Autodesk Inventor part; units mm, degrees
ref_plane "YZ Plane" through (0, 0, 0) normal (1, 0, 0) x (0, 1, 0)
ref_plane "XZ Plane" through (0, 0, 0) normal (0, 1, 0) x (-1, 0, 0)
ref_plane "XY Plane" through (0, 0, 0) normal (0, 0, 1) x (1, 0, 0)
sketch "Sketch1" plane through (0, 0, 0) normal (0, 0, 1) x (1, 0, 0)
  line L0 (-22.85, 10.65) -> (22.85, 10.65)
  line L1 (22.85, 10.65) -> (22.85, -10.65)
  line L2 (22.85, -10.65) -> (-22.85, -10.65)
  line L3 (-22.85, -10.65) -> (-22.85, 10.65)
  line L4 (0, 0) -> (0, 10.65) construction
  line L5 (0, 0) -> (0, -10.65) construction
  line L6 (0, 0) -> (22.85, 0) construction
  line L7 (0, 0) -> (-22.85, 0) construction
  dimension "d0" = 45.7
  dimension "d1" = 21.3
extrude "Extrusion1" add sketch "Sketch1" along normal blind 1.75
sketch "Sketch2" plane through (0, 0, 1.75) normal (0, 0, 1) x (1, 0, 0)
  line L0 (22.85, 10.65) -> (22.85, -10.65)
  line L1 (-22.85, 10.65) -> (22.85, 10.65)
  line L2 (22.85, -10.65) -> (-22.85, -10.65)
  point P0 (-20.35, -8.15)
  point P1 (20.35, 8.15)
  dimension "d4" = 2.5
  dimension "d5" = 2.5
  dimension "d6" = 2.5
  dimension "d7" = 2.5
hole "Hole1" at (-20.35, -8.15, 1.75) at (20.35, 8.15, 1.75) direction (0, 0, -1) diameter 3.1 end through all
properties part number "Parallax_Ping_PCB" material "Phenolic"
Geometry check sheet. Reference: the model listing, model coordinates, mm. Give positions to 0.01 mm unless a question says otherwise; leave off trailing zeros. Order: outer loops, then holes, each group sorted by start corner. A loop starts at its lowest first (then second) coordinate and runs counter-clockwise, first axis right, second up. Notation, with made-up numbers: (10.25, 32) - (66.25, 32) arc R24 cw to (66.25, 55) - close; hole circle Ø10 at (-9.5, -18). An arc over 180 degrees is marked (long way). Use one line per item in the form item = value.
1) Sectioned sample at B-B (z = 0.4). Record the boundary of the cut face in (x, y).
Working result:
outline = (-22.85, -10.65) - (22.85, -10.65) - (22.85, 10.65) - (-22.85, 10.65) - close; hole circle Ø3.1 at (-20.35, -8.15); hole circle Ø3.1 at (20.35, 8.15)
2) Sectioned sample at C-C (x = 20.35). Record the boundary of the cut face in (y, z), and give its area (4 significant figures).
Working result:
outline = (-10.65, 0) - (6.6, 0) - (6.6, 1.75) - (-10.65, 1.75) - close; (9.7, 0) - (10.65, 0) - (10.65, 1.75) - (9.7, 1.75) - close
area = 31.85 mm^2
3) Draft check along Y on faces 1 (the face through (0, 10.65, 1)), 2 (the face through (0, -10.65, 1)), 3 (the face through (21.29, 9.38, 0.86)). Enter one of: released by +Y, released by -Y, zero draft, split by the parting line, or undercut.
Working result:
face_1 = released by +Y
face_2 = released by -Y
face_3 = undercut
4) Material ranges on probe 1 along X at (y, z) = (-8.15, 0.9); probe 2 along X at (y, z) = (8.15, 0.95); probe 3 along Y at (x, z) = (20.35, 1), recorded low to high. Write a range as from..to.
Working result:
probe_1 = -22.85..-21.9, -18.8..22.85
probe_2 = -22.85..18.8, 21.9..22.85
probe_3 = -10.65..6.6, 9.7..10.65
5) Sectioned sample at A-A (y = -8.15). Record the boundary of the cut face in (x, z), and give its area (4 significant figures).
Working result:
outline = (-22.85, 0) - (-21.9, 0) - (-21.9, 1.75) - (-22.85, 1.75) - close; (-18.8, 0) - (22.85, 0) - (22.85, 1.75) - (-18.8, 1.75) - close
area = 74.55 mm^2
